Here's the drawing with two shaded views (mm, measured from the low corner). I have some questions. Round coordinates to 2 decimals unless told otherwise and drop trailing zeros. Order: outer loops, then holes, each group sorted by start corner. A loop starts at its lowest first (then second) coordinate and runs counter-clockwise, first axis right, second up.
Q1. If I drill on line 1 (Z direction, x = 27, y = 11.55); line 2 (Z direction, x = 27, y = 4.75); line 3 (X direction, y = 11.4, z = 60), over which ranges is the centre line in solid material (lowest first)?
Q2. If we section it at D-D (y = 11.25): Please give me the cut outline in (x, z), plus the area to 3 significant figures.
Q3. If we section it at B-B (z = 80): Please give me the cut outline in (x, y).
Q4. Will these pins go through, and if not, where does the flat tip stop? P1, Ø4, axis at y = 2, z = 53, coming from the +X side; P2, Ø6, axis at y = 9, z = 43, coming from the +X side; P3, Ø4, axis at x = 28.5, z = 30.5, coming from the +Y side; P4, Ø12, axis at x = 27, z = 60, coming from the +Y side.
Q5. If we section it at C-C (y = 1): Please give me the cut outline in (x, z) (1 decimal), plus the area to 3 significant figures.
Q6. If we section it at A-A (x = 27): Please give me the cut outline in (y, z).
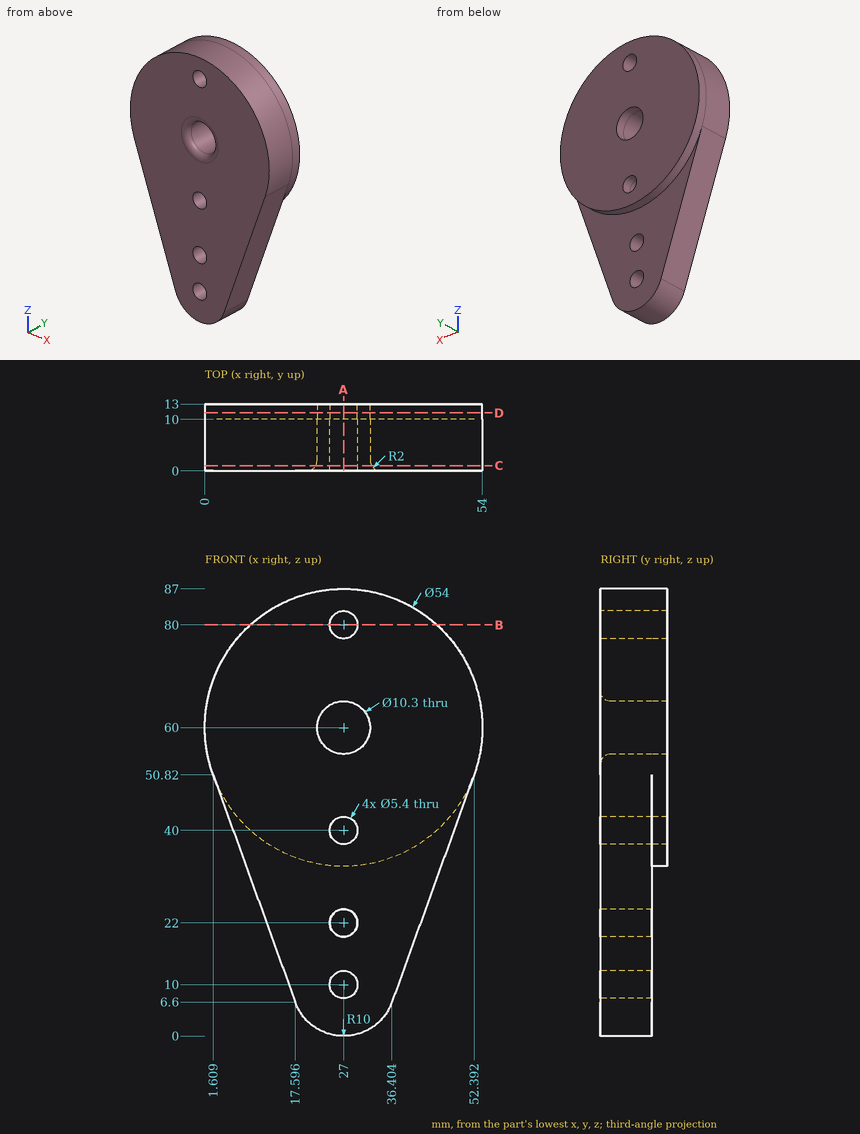
Solution:
1. line 1: z = 33 to 37.3, 42.7 to 54.85, 65.15 to 77.3, 82.7 to 87
1. line 2: z = 0 to 7.3, 12.7 to 19.3, 24.7 to 37.3, 42.7 to 54.85, 65.15 to 77.3, 82.7 to 87
1. line 3: x = 0 to 21.85, 32.15 to 54
2. outline: circle Ø54 at (27, 60); hole circle Ø10.3 at (27, 60); hole circle Ø5.4 at (27, 40); hole circle Ø5.4 at (27, 80)
2. area: 2,160 mm2
3. outline: (8.86, 0) - (24.3, 0) - (24.3, 13) - (8.86, 13) - close; (29.7, 0) - (45.14, 0) - (45.14, 13) - (29.7, 13) - close
4. P1: stops at x = 53.53
4. P2: stops at x = 50.65
4. P3: stops at y = 10
4. P4: stops at y = 13
5. outline: (1.6, 50.8) - (17.6, 6.6) arc R10 ccw to (36.4, 6.6) - (52.4, 50.8) arc R27 ccw (long way) to start; hole circle Ø10.8 at (27, 60); hole circle Ø5.4 at (27, 10); hole circle Ø5.4 at (27, 22); hole circle Ø5.4 at (27, 40); hole circle Ø5.4 at (27, 80)
5. area: 3,080 mm2
6. outline: (0, 0) - (10, 0) - (10, 7.3) - (0, 7.3) - close; (0, 12.7) - (10, 12.7) - (10, 19.3) - (0, 19.3) - close; (0, 24.7) - (10, 24.7) - (10, 33) - (13, 33) - (13, 37.3) - (0, 37.3) - close; (0, 42.7) - (13, 42.7) - (13, 54.85) - (2, 54.85) arc R2 ccw to (0, 52.85) - close; (0, 67.15) arc R2 ccw to (2, 65.15) - (13, 65.15) - (13, 77.3) - (0, 77.3) - close; (0, 82.7) - (13, 82.7) - (13, 87) - (0, 87) - close
